Part model, mm, in its own coordinate system. A direction names the side the tool comes from. Give positions to 0.01 mm unless a question says otherwise; leave off trailing zeros. Loops run counter-clockwise (first coordinate to the right, second up) from the corner with the lowest first, then second, coordinate; pieces in that order, holes last. Notation, with made-up numbers: M 46.25,-19 L 51.25,-19 A19 cw 51.25,4 Z; hole C -29.75,-34 d11. An arc over 180 degrees is marked long. Answer in a Markdown table with one row per item.
Autodesk Inventor part; units mm, degrees
ref_plane "YZ Plane" through (0, 0, 0) normal (1, 0, 0) x (0, 1, 0)
ref_plane "XZ Plane" through (0, 0, 0) normal (0, 1, 0) x (-1, 0, 0)
ref_plane "XY Plane" through (0, 0, 0) normal (0, 0, 1) x (1, 0, 0)
sketch "Sketch1" plane through (0, 0, 0) normal (0, 0, 1) x (1, 0, 0)
  circle A0 centre (0, 0) radius 1 construction
  circle A1 centre (2.5, 0) radius 1 construction
  circle A2 centre (-2.5, 0) radius 1 construction
  circle A3 centre (-1.25, 2) radius 1 construction
  circle A4 centre (1.25, 2) radius 1 construction
  line L0 (-4, 2.5) -> (4, 2.5)
  line L1 (4, 2.5) -> (4, -0.5)
  line L2 (4, -0.5) -> (-4, -0.5)
  line L3 (-4, -0.5) -> (-4, 2.5)
  line L4 (-4, 2.5) -> (4, -0.5) construction
  line L5 (4, 2.5) -> (-4, -0.5) construction
  line L6 (6, 4.5) -> (-6, 4.5)
  line L7 (-6, 4.5) -> (-6, -2.5)
  line L8 (-6, -2.5) -> (6, -2.5)
  line L9 (6, -2.5) -> (6, 4.5)
  point P0 (0, 1)
  point P1 (0, 1)
  dimension "d0" = 2
  dimension "d1" = 2.5
  dimension "d2" = 2.5
  dimension "d3" = 1.25
  dimension "d4" = 2
  dimension "d5" = 1.25
  dimension "d6" = 1
  dimension "d7" = 3
  dimension "d8" = 8
  dimension "d9" = 2
extrude "Extrusion1" add sketch "Sketch1" along normal blind 4
sketch "Sketch2" plane through (-6, 4.5, 0) normal (0, 1, 0) x (1, 0, 0)
  line L0 (2, 0) -> (2, -4)
  line L1 (10, 0) -> (10, -4)
  line L2 (4, -4) -> (8, 0) construction
  line L3 (12, -4) -> (0, -4)
  line L4 (12, 0) -> (0, 0)
  line L5 (3.7, -4) -> (7.7, 0)
  line L6 (10, 0) -> (2, 0)
  line L7 (4.3, -4) -> (8.3, 0)
  line L8 (3.7, -4) -> (4.3, -4)
  line L9 (7.7, 0) -> (8.3, 0)
  point P0 (6, 0)
  dimension "d12" = 2
  dimension "d13" = 2
  dimension "d15" = 0.3
  dimension "d16" = 0.3
extrude "Extrusion2" cut sketch "Sketch2" against normal blind 4 contours L4 L7 L3 L5
chamfer "Chamfer1" distance 0.75 angle 45 2 edges at (0.3, 4.5, 2) (-0.3, 4.5, 2)
fillet "Fillet1" radius 0.75 4 edges at (-4, -0.5, 2) (-4, 2.5, 2) (4, 2.5, 2) (4, -0.5, 2)
fillet "Fillet1" radius 0.75 2 edges at (-6, 4.5, 2) (6, 4.5, 2)
equation "\"d13\" = d12"
equation "\"d16\" = d15"
properties part number "Cable Clip v1"
(1) Saw through at C-C (x = -1.25). Write the cut outline in (y, z), plus the area to 3 significant figures.
Recorded:
| item | result |
|---|---|
| outline | M -2.5,0 L -0.5,0 L -0.5,4 L -2.5,4 Z; M 2.5,0 L 4.5,0 L 4.5,1.89 L 3.75,2.95 L 2.5,2.95 Z; M 2.5,3.55 L 3.75,3.55 L 4.07,4 L 2.5,4 Z |
| area | 14.1 mm^2 |
(2) Saw through at A-A (y = 3.5). Write the cut outline in (x, z).
Recorded:
| item | result |
|---|---|
| outline | M -6,0 L 1.7,0 L -2.3,4 L -6,4 Z; M -1.7,4 L 2.3,0 L 6,0 L 6,4 Z |
(3) Saw through at B-B (x = -2.5). Write the cut outline in (y, z), plus the area to 3 significant figures.
Recorded:
| item | result |
|---|---|
| outline | M -2.5,0 L -0.5,0 L -0.5,4 L -2.5,4 Z; M 2.5,0 L 4.5,0 L 4.5,3.14 L 3.89,4 L 2.5,4 Z |
| area | 15.7 mm^2 |
(4) Pull direction X, two halves, no side cores. Call faces 1 (the face through (-0.3, 3.1, 2)), 2 (the face through (-6, 1, 2)), 3 (the face through (6, 1, 2)): +X half, -X half, draft (parallel to the pull), parting line (faces both ways), or undercut.
Recorded:
| item | result |
|---|---|
| face 1 | undercut |
| face 2 | -X half |
| face 3 | +X half |
(5) Which spindle directions (+Z, -Z, +X, -X, +Y, -Y) get a long thin tool onto all of the face, cutting with end or side? Do faces 4 (the face through (0, -0.5, 2)), 5 (the face through (0, -1, 4)), 6 (the face through (-0.86, 4.12, 2.04)). Say none if no direction does.
Recorded:
| item | result |
|---|---|
| face 4 | +Z, -Z |
| face 5 | +Z, +X, -X, +Y, -Y |
| face 6 | +Y |
(6) Drill centre lines: line 1 along Y through (x, z) = (-3, 3.3); line 2 along X through (y, z) = (0.25, 0.35); line 3 along Y through (x, z) = (-0.5, 1.85). Where is each one in solid material? Low to high.
Recorded:
| item | result |
|---|---|
| line 1 | y = -2.5 to -0.5, 2.5 to 4.5 |
| line 2 | x = -6 to -4, 4 to 6 |
| line 3 | y = -2.5 to -0.5, 2.5 to 4 |
(7) Saw through at D-D (y = 0.5). Write the cut outline in (x, z).
Recorded:
| item | result |
|---|---|
| outline | M -6,0 L -4,0 L -4,4 L -6,4 Z; M 4,0 L 6,0 L 6,4 L 4,4 Z |
